from build123d import *

# Parameters (mm, degrees)
Y_KSEKLIK_EKSTR_ZYON1_DEPTH = 4
PAH2_SIZE                   = 0.65
PAH7_SIZE                   = 0.3
PAH8_SIZE                   = 0.3
IZIM2_W                     = 0.65
IZIM2_H                     = 0.45
Y_KSEKLIK_EKSTR_ZYON2_DEPTH = 2.75


with BuildPart() as part:
    # Çizim1 → Yükseklik-Ekstrüzyon1 (new body)
    with BuildSketch(Plane.XY):
        Polygon((0, 0), (5, 0), (5, 5.8), (4, 6.8), (1, 6.8), (0, 5.8), align=None)
    extrude(amount=Y_KSEKLIK_EKSTR_ZYON1_DEPTH)

    # Pah2
    pah2_edges = [part.edges().sort_by_distance(p)[0] for p in [
        (5, 2.9, 4),
        (0, 2.9, 4),
    ]]
    chamfer(pah2_edges, length=PAH2_SIZE)

    # Pah3
    # the kernel refuses this chamfer: 0.65 mm, written as the material it takes off along each edge
    with BuildSketch(Plane(origin=(0, 5.8, -0.733571059), x_dir=(-0.033908675640741216, -0.9994249355085608, 0), z_dir=(0, 0, 1))) as pah3_piece_1:
        with BuildLine():
            Line((0.293428424, 0), (-0.221071103, 0.192945089))
            Line((-0.221071103, 0.192945089), (-0.229946503, 0.183446285))
            ThreePointArc((-0.229946503, 0.183446285), (-0.116014483, 0.090608776), (-0.0088754, -0.009498804))
            Line((-0.0088754, -0.009498804), (0.000440813, -0.012992524))
            ThreePointArc((0.000440813, -0.012992524), (0.146986333, -0.0080205), (0.293869236, -0.012992524))
            Line((0.293869236, -0.012992524), (0.293428424, 0))
        make_face()
    extrude(amount=4.817142118, mode=Mode.SUBTRACT)

    # Pah4
    # the kernel refuses this chamfer: 0.65 mm, written as the material it takes off along each edge
    with BuildSketch(Plane(origin=(5, 5.8, -0.733571059), x_dir=(0.03390867564074173, -0.9994249355085608, 0), z_dir=(0, 0, 1))) as pah4_piece_1:
        with BuildLine():
            Line((0.293428424, 0), (-0.221071103, -0.192945089))
            Line((-0.221071103, -0.192945089), (-0.229946503, -0.183446285))
            ThreePointArc((-0.229946503, -0.183446285), (-0.116014483, -0.090608776), (-0.0088754, 0.009498804))
            Line((-0.0088754, 0.009498804), (0.000440813, 0.012992524))
            ThreePointArc((0.000440813, 0.012992524), (0.146986333, 0.0080205), (0.293869236, 0.012992524))
            Line((0.293869236, 0.012992524), (0.293428424, 0))
        make_face()
    extrude(amount=4.817142118, mode=Mode.SUBTRACT)

    # Pah7
    pah7_edges = [part.edges().sort_by_distance(p)[0] for p in [
        (0.65, 3.225, 4),
    ]]
    chamfer(pah7_edges, length=PAH7_SIZE)

    # Pah8
    pah8_edges = [part.edges().sort_by_distance(p)[0] for p in [
        (4.35, 3.225, 4),
    ]]
    chamfer(pah8_edges, length=PAH8_SIZE)

    # Çizim2 → Yükseklik-Ekstrüzyon2 (add)
    with BuildSketch(Plane.XZ):
        with Locations((1.25, 2.825)):
            Rectangle(IZIM2_W, IZIM2_H)
        with Locations((3.75, 2.825)):
            Rectangle(IZIM2_W, IZIM2_H)
    extrude(amount=Y_KSEKLIK_EKSTR_ZYON2_DEPTH)


solid = part.part
Design review of the part built by this model. Coordinates are the model's own, in mm. Round coordinates to 2 decimals unless told otherwise and drop trailing zeros. Write each loop counter-clockwise with the first axis right and the second up, starting at its lowest first coordinate (ties: lowest second). Pieces come first, ordered by that corner, then holes. Notation, with made-up numbers: (72.5, 64) - (103.5, 64) arc R28 ccw to (103.5, 98) - close; hole circle Ø10 at (66, 19). An arc over 180 degrees is marked (long way). Use a Markdown table: item, result. Add a question column.
1. We need section C-C (x = 3.15). State the section outline as (y, z) points, then the cut area to 3 significant figures.
2. We need section D-D (y = 2.75). State the section outline as (x, z) points, then the cut area to 3 significant figures.
3. We need section B-B (z = 3.25). State the section outline as (x, y) points, then the cut area to 3 significant figures.
4. Clearance check with flat-ended pins moving along their axes: pin 1 (0.5 mm diameter, centred on y = -1.5, z = 3, fed in from -X) (3 decimals); pin 2 (2 mm diameter, centred on x = 2, z = 1, fed in from -Y); pin 3 (0.5 mm diameter, centred on y = -1, z = 2.5, fed in from +X) (3 decimals). State where each tip first meets the part, or that it passes through.
5. We need section A-A (y = -1.25). State the section outline as (x, z) points (3 decimals).
6. Wall thickness on probe 1 along X at (y, z) = (-0.25, 2.7) (3 decimals); probe 2 along Y at (x, z) = (1.9, 3.15); probe 3 along Y at (x, z) = (4.3, 0.3): over which ranges is each line inside the solid? List them lowest first.
Output:
| question | item | result |
|---|---|---|
| 1 | outline | (0, 0) - (6.8, 0) - (6.8, 4) - (0, 4) - close |
| 1 | area | 27.2 mm2 |
| 2 | outline | (0, 0) - (5, 0) - (5, 3.35) - (4.56, 3.79) - (4.05, 4) - (0.95, 4) - (0.44, 3.79) - (0, 3.35) - close |
| 2 | area | 19.5 mm2 |
| 3 | outline | (0, 0) - (5, 0) - (5, 5.53) - (4.81, 5.99) - (4, 6.8) - (1, 6.8) - (0.19, 5.99) - (0, 5.53) - close |
| 3 | area | 32.9 mm2 |
| 4 | pin 1 | stops at x = 0.925 |
| 4 | pin 2 | stops at y = 0 |
| 4 | pin 3 | stops at x = 4.075 |
| 5 | outline | (0.925, 2.6) - (1.575, 2.6) - (1.575, 3.05) - (0.925, 3.05) - close; (3.425, 2.6) - (4.075, 2.6) - (4.075, 3.05) - (3.425, 3.05) - close |
| 6 | probe 1 | x = 0.925 to 1.575, 3.425 to 4.075 |
| 6 | probe 2 | y = 0 to 6.8 |
| 6 | probe 3 | y = 0 to 6.5 |
